from build123d import *

# Parameters (mm, degrees)
SKETCH1_W           = 101.6
SKETCH1_H           = 101.6
BOSS_EXTRUDE1_DEPTH = 19.05
SKETCH2_R           = 8.001
CUT_EXTRUDE1_DEPTH  = 19.05
SKETCH3_R           = 1.651
CUT_EXTRUDE2_DEPTH  = 19.05
SKETCH4_R           = 1.651
CUT_EXTRUDE3_DEPTH  = 19.05


with BuildPart() as part:
    # Sketch1 → Boss-Extrude1 (new body)
    with BuildSketch(Plane.XY):
        Rectangle(SKETCH1_W, SKETCH1_H)
    extrude(amount=BOSS_EXTRUDE1_DEPTH)

    # Sketch2 → Cut-Extrude1 (cut)
    with BuildSketch(Plane.XY.offset(19.05)):
        with Locations((0, 25.4)):
            Circle(SKETCH2_R)
    extrude(amount=-CUT_EXTRUDE1_DEPTH, mode=Mode.SUBTRACT)

    # Sketch3 → Cut-Extrude2 (cut)
    with BuildSketch(Plane.XY.offset(19.05)):
        with Locations((-38.1, -40.767)):
            Circle(SKETCH3_R)
    extrude(amount=-CUT_EXTRUDE2_DEPTH, mode=Mode.SUBTRACT)

    # Sketch4 → Cut-Extrude3 (cut)
    with BuildSketch(Plane.XY.offset(19.05)):
        with Locations((-38.1, 40.767)):
            Circle(SKETCH4_R)
        with Locations((38.1, 40.767)):
            Circle(SKETCH4_R)
        with Locations((38.1, -40.767)):
            Circle(SKETCH4_R)
    extrude(amount=-CUT_EXTRUDE3_DEPTH, mode=Mode.SUBTRACT)


solid = part.part
Can you work these out from the model? Positions are in its coordinate system, mm. Coordinates: 2 decimals unless noted, no trailing zeros. Write each loop counter-clockwise with the first axis right and the second up, starting at its lowest first coordinate (ties: lowest second). Pieces come first, ordered by that corner, then holes. Notation, with made-up numbers: (-6, -4.5) -> (-1, -4.5) arc R4 ccw to (-1, 0.5) -> close; hole circle Ø11 at (28.5, 65). An arc over 180 degrees is marked (long way). Write each question's results on one line, items separated by ' | '. Start each with the question number.
Item 1: If we section it at C-C, the plane x = 0: Write out the boundary of the cut face in (y, z).
Item 2: Thinking about a two-plate mould opening in X: for faces 1 (the flat face through (-1, 1, 0)), 2 (the flat face through (50.8, -1, 9)), 3 (the flat face through (-50.8, -1, 9)), 4 (the cylindrical face through (-36.575, 40.135, 9.658)), which applies, released by +X, released by -X, zero draft, split by the parting line, or undercut?
Item 3: If we section it at D-D, the plane z = 13: Write out the boundary of the cut face in (x, y).
Item 4: If we section it at B-B, the plane y = 25.4: Write out the boundary of the cut face in (x, z).
Item 5: Please list where these lines run through material, in increasing order: probe 1 along Y at (x, z) = (-38.1, 13.75); probe 2 along X at (y, z) = (-40.5, 10.75); probe 3 along X at (y, z) = (-42, 15.5).
Item 6: If we section it at A-A, the plane x = -38.1: Write out the boundary of the cut face in (y, z), and give its area (3 significant figures).
Item 7: I'm going to push a flat-ended pin straight in: P1, Ø2.5, axis at x = -38.1, y = -40.767, coming from the -Z side. Where does the tip first touch, or does it pass through?
Answer block:
1) outline: (-50.8, 0) -> (17.4, 0) -> (17.4, 19.05) -> (-50.8, 19.05) -> close; (33.4, 0) -> (50.8, 0) -> (50.8, 19.05) -> (33.4, 19.05) -> close
2) face 1: zero draft | face 2: released by +X | face 3: released by -X | face 4: undercut
3) outline: (-50.8, -50.8) -> (50.8, -50.8) -> (50.8, 50.8) -> (-50.8, 50.8) -> close; hole circle Ø3.3 at (-38.1, -40.77); hole circle Ø3.3 at (-38.1, 40.77); hole circle Ø16 at (0, 25.4); hole circle Ø3.3 at (38.1, -40.77); hole circle Ø3.3 at (38.1, 40.77)
4) outline: (-50.8, 0) -> (-8, 0) -> (-8, 19.05) -> (-50.8, 19.05) -> close; (8, 0) -> (50.8, 0) -> (50.8, 19.05) -> (8, 19.05) -> close
5) probe 1: -50.8 to -42.42, -39.12 to 39.12, 42.42 to 50.8 | probe 2: -50.8 to -39.73, -36.47 to 36.47, 39.73 to 50.8 | probe 3: -50.8 to -39.2, -37 to 37, 39.2 to 50.8
6) outline: (-50.8, 0) -> (-42.42, 0) -> (-42.42, 19.05) -> (-50.8, 19.05) -> close; (-39.12, 0) -> (39.12, 0) -> (39.12, 19.05) -> (-39.12, 19.05) -> close; (42.42, 0) -> (50.8, 0) -> (50.8, 19.05) -> (42.42, 19.05) -> close | area: 1,810 mm²
7) P1: through
